Build history of the part. All positions in model axes, mm. Face numbers are marked on the shaded views. A direction names the side the tool comes from. Round coordinates to 2 decimals unless told otherwise and drop trailing zeros. Write each loop counter-clockwise with the first axis right and the second up, starting at its lowest first coordinate (ties: lowest second). Pieces come first, ordered by that corner, then holes.
1) Flat gauge pins, fed straight in: pin 1 (12 mm diameter, centred on x = 30.5, y = 23.5, fed in from -Z); pin 2 (6 mm diameter, centred on y = 38.5, z = -18, fed in from +X); pin 3 (25 mm diameter, centred on x = -54, z = -10.5, fed in from +Y); pin 4 (12.5 mm diameter, centred on x = -30, z = 0, fed in from +Y). Where does each tip first touch, or does it go through?
2) Wall check: probe 1 along Y at (x, z) = (-23, -4.5); probe 2 along Y at (x, z) = (21.5, -4.5); probe 3 along Z at (x, y) = (-36.5, 43.5). Give the ranges that are in metal, low to high.
3) Saw through at D-D (y = 90). Write the cut outline in (x, z), plus the area to 3 significant figures.
4) Which spindle directions (+Z, -Z, +X, -X, +Y, -Y) get a long thin tool onto all of the face, cutting with end or side? Do the marked faces 4 and 5. Say none if no direction does.
5) Saw through at A-A (x = -100). Write the cut outline in (y, z).
6) Saw through at B-B (y = -4). Write the cut outline in (x, z), plus the area to 3 significant figures.
7) Saw through at C-C (x = -30). State how many separate pieces and enclosed holes the cut face has, plus the area to 3 significant figures.
8) Pull direction Z, two halves, no side cores. Call the marked faces 1, 2 and 3: +Z half, -Z half, draft (parallel to the pull), parting line (faces both ways), or undercut.
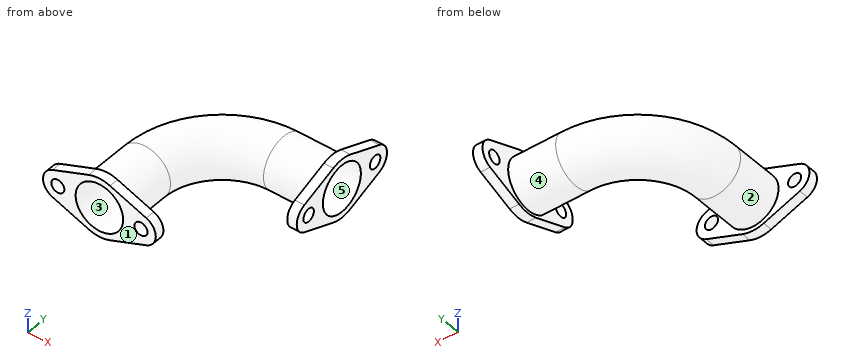
from build123d import *

# Parameters (mm, degrees)
SWEEP4_PROFILE_R     = 21.5
SKETCH21_R           = 5.5
BOSS_EXTRUDE5_DEPTH  = 8
SKETCH24_R           = 5.5
SKETCH24_R_2         = 17.5
BOSS_EXTRUDE6_DEPTH  = 8
SKETCH26_R           = 20
CUT_EXTRUDE1_DEPTH   = 48
SKETCH27_R           = 20
CUT_EXTRUDE2_DEPTH   = 48
CUT_SWEEP1_PROFILE_R = 20


with BuildPart() as part:
    # Sweep4: sweep along a path in Sketch1
    with BuildLine(Plane.XY) as sweep4_path:
        Line((40, 65), (0, 65))
        ThreePointArc((0, 65), (-45.961940777, 45.961940777), (-65, 0))
        Line((-65, 0), (-65, -40))
    # Sweep4 profile (on start of the path) → Sweep4 (sweep)
    with BuildSketch(Plane(origin=(40, 65, 0), x_dir=(0, 0, -1), z_dir=(-1, 0, 0))):
        Circle(SWEEP4_PROFILE_R)
    sweep(path=sweep4_path.line)

    # Sketch21 → Boss-Extrude5 (add)
    with BuildSketch(Plane.XZ.offset(40)):
        with BuildLine():
            Line((-104.464285714, 11.67562217), (-73.928571429, 23.35124434))
            ThreePointArc((-73.928571429, 23.35124434), (-65, 25), (-56.071428571, 23.35124434))
            Line((-56.071428571, 23.35124434), (-25.535714286, 11.67562217))
            ThreePointArc((-25.535714286, 11.67562217), (-17.5, 0), (-25.535714286, -11.67562217))
            Line((-25.535714286, -11.67562217), (-56.071428571, -23.35124434))
            ThreePointArc((-56.071428571, -23.35124434), (-65, -25), (-73.928571429, -23.35124434))
            Line((-73.928571429, -23.35124434), (-104.464285714, -11.67562217))
            ThreePointArc((-104.464285714, -11.67562217), (-112.5, 0), (-104.464285714, 11.67562217))
        make_face()
        with Locations((-100, 0)):
            Circle(SKETCH21_R, mode=Mode.SUBTRACT)
        with Locations((-30, 0)):
            Circle(SKETCH21_R, mode=Mode.SUBTRACT)
    extrude(amount=BOSS_EXTRUDE5_DEPTH)

    # Sketch24 → Boss-Extrude6 (add)
    with BuildSketch(Plane(origin=(40, 0, 0), x_dir=(0, 0, -1), z_dir=(1, 0, 0))):
        with BuildLine():
            Line((-12.573810861, 26.563231974), (-24.249433031, 57.09894626))
            ThreePointArc((-24.249433031, 57.09894626), (-25.898188691, 66.027517688), (-24.249433031, 74.956089117))
            Line((-24.249433031, 74.956089117), (-12.573810861, 105.491803403))
            ThreePointArc((-12.573810861, 105.491803403), (-0.898188691, 113.527517688), (10.77743348, 105.491803403))
            Line((10.77743348, 105.491803403), (22.45305565, 74.956089117))
            ThreePointArc((22.45305565, 74.956089117), (24.101811309, 66.027517688), (22.45305565, 57.09894626))
            Line((22.45305565, 57.09894626), (10.77743348, 26.563231974))
            ThreePointArc((10.77743348, 26.563231974), (-0.898188691, 18.527517688), (-12.573810861, 26.563231974))
        make_face()
        with Locations(Location((-0.898188691, 31.027517688, 0), (0, 0, 90))):
            Circle(SKETCH24_R, mode=Mode.SUBTRACT)
        with Locations((-0.898188691, 66.027517688)):
            Circle(SKETCH24_R_2, mode=Mode.SUBTRACT)
        with Locations(Location((-0.898188691, 101.027517688, 0), (0, 0, 90))):
            Circle(SKETCH24_R, mode=Mode.SUBTRACT)
    extrude(amount=BOSS_EXTRUDE6_DEPTH)

    # Sketch26 → Cut-Extrude1 (cut)
    with BuildSketch(Plane.XZ.offset(48)):
        with Locations((-65, 0)):
            Circle(SKETCH26_R)
    extrude(amount=-CUT_EXTRUDE1_DEPTH, mode=Mode.SUBTRACT)

    # Sketch27 → Cut-Extrude2 (cut)
    with BuildSketch(Plane(origin=(48, 0, 0), x_dir=(0, 0, -1), z_dir=(1, 0, 0))):
        with Locations(Location((-0.898188691, 66.027517688, 0), (0, 0, 90))):
            Circle(SKETCH27_R)
    extrude(amount=-CUT_EXTRUDE2_DEPTH, mode=Mode.SUBTRACT)

    # Cut-Sweep1: sweep along a path in Sketch28
    with BuildLine(Plane.XY) as cut_sweep1_path:
        ThreePointArc((0, 65), (-45.961940777, 45.961940777), (-65, 0))
    # Cut-Sweep1 profile (on start of the path) → Cut-Sweep1 (sweep, cut)
    with BuildSketch(Plane(origin=(0, 65, 0), x_dir=(0, -1, 0), z_dir=(-1, 0, 0))):
        Circle(CUT_SWEEP1_PROFILE_R)
    sweep(path=cut_sweep1_path.line, mode=Mode.SUBTRACT)


solid = part.part
Evaluation:
1. pin 1: passes through
1. pin 2: stops at x = 48
1. pin 3: stops at y = 74.5
1. pin 4: stops at y = 83.18
2. probe 1: y = -48 to -40, 37.48 to 39.27, 81.3 to 82.89
2. probe 2: y = 43.98 to 46.77, 85.29 to 86.02
2. probe 3: z = -19.87 to -18.23, 18.23 to 19.87
3. outline: (40, -16.7) - (48, -16.7) - (48, 18.5) - (40, 18.5) - close
3. area: 282 mm2
4. face 4: none
4. face 5: +X
5. outline: (-48, -13.38) - (-40, -13.38) - (-40, -5.5) - (-48, -5.5) - close; (-48, 5.5) - (-40, 5.5) - (-40, 13.38) - (-48, 13.38) - close
6. outline: circle Ø43 at (-65, 0); hole circle Ø40 at (-65, 0)
6. area: 196 mm2
7. separate pieces: 3
7. enclosed holes: 1
7. area: 354 mm2
8. face 1: draft
8. face 2: parting line
8. face 3: undercut
